CAD build for the part. Positions are in the model's coordinates, mm. A direction names the side the tool comes from. Round coordinates to 2 decimals unless told otherwise and drop trailing zeros. Write each loop counter-clockwise with the first axis right and the second up, starting at its lowest first coordinate (ties: lowest second). Pieces come first, ordered by that corner, then holes. Notation, with made-up numbers: M 27.5,-24 L 60.5,-24 A20 cw 60.5,10 Z; hole C 30.25,48 d4. An arc over 180 degrees is marked long. Write each question's results on one line, items separated by ' | '. Start each with the question number.
```python
from build123d import *

# Parameters (mm, degrees)
SKETCH1_W                = 44
SKETCH1_H                = 25
BOSS_EXTRUDE1_DEPTH      = 4.5
SKETCH2_W                = 44
SKETCH2_H                = 6
BOSS_EXTRUDE2_DEPTH      = 22
SKETCH3_R                = 1.6
SKETCH3_R_2              = 2.1
SKETCH3_R_3              = 3.1
SKETCH3_R_4              = 6.05
CUT_EXTRUDE1_DEPTH       = 34.529837459
SKETCH4_R                = 6.1
CUT_EXTRUDE2_DEPTH       = 0.7
SKETCH5_R                = 4.1
CUT_EXTRUDE3_DEPTH       = 0.5
SKETCH6_R                = 3.1
CUT_EXTRUDE4_DEPTH       = 0.4
CHAMFER4_SIZE            = 3
CHAMFER5_SIZE            = 2
CHAMFER6_SIZE            = 1.5
CHAMFER4_OF_MIRROR1_SIZE = 3
CHAMFER5_OF_MIRROR1_SIZE = 2
CHAMFER6_OF_MIRROR1_SIZE = 1.5
CUT_EXTRUDE5_DEPTH       = 43.558782877


with BuildPart() as part:
    # Sketch1 → Boss-Extrude1 (new body)
    with BuildSketch(Plane.XY):
        Rectangle(SKETCH1_W, SKETCH1_H)
    extrude(amount=BOSS_EXTRUDE1_DEPTH)

    # Sketch2 → Boss-Extrude2 (add)
    with BuildSketch(Plane.XY.offset(4.5)):
        with Locations((0, 9.5)):
            Rectangle(SKETCH2_W, SKETCH2_H)
    extrude(amount=BOSS_EXTRUDE2_DEPTH)

    # Sketch3 → Cut-Extrude1 (cut, through all)
    with BuildSketch(Plane.XY.offset(4.5)):
        with Locations((-14, -8.5)):
            Circle(SKETCH3_R)
        with Locations((-14, 0.682507664)):
            Circle(SKETCH3_R_2)
        with Locations((-3.234639789, -4.5)):
            Circle(SKETCH3_R_3)
        with Locations((12.315992983, -2.743651106)):
            Circle(SKETCH3_R_4)
    cut_extrude1 = extrude(amount=-CUT_EXTRUDE1_DEPTH, mode=Mode.SUBTRACT)

    # Sketch4 → Cut-Extrude2 (cut)
    with BuildSketch(Plane.XY.offset(4.5)):
        with Locations((-3.234639789, -4.5)):
            Circle(SKETCH4_R)
    cut_extrude2 = extrude(amount=-CUT_EXTRUDE2_DEPTH, mode=Mode.SUBTRACT)

    # Sketch5 → Cut-Extrude3 (cut)
    with BuildSketch(Plane.XY.offset(4.5)):
        with Locations((-14, 0.682507664)):
            Circle(SKETCH5_R)
    cut_extrude3 = extrude(amount=-CUT_EXTRUDE3_DEPTH, mode=Mode.SUBTRACT)

    # Sketch6 → Cut-Extrude4 (cut)
    with BuildSketch(Plane.XY.offset(4.5)):
        with Locations((-14, -8.5)):
            Circle(SKETCH6_R)
    cut_extrude4 = extrude(amount=-CUT_EXTRUDE4_DEPTH, mode=Mode.SUBTRACT)

    # Chamfer4
    chamfer4_edges = [part.edges().sort_by_distance(p)[0] for p in [
        (-6.334639789, -4.5, 3.8),
    ]]
    chamfer(chamfer4_edges, length=CHAMFER4_SIZE - 0.0001)  # a hair under: the kernel refuses the full size

    # Chamfer5
    chamfer5_edges = [part.edges().sort_by_distance(p)[0] for p in [
        (-16.1, 0.682507664, 4),
    ]]
    chamfer(chamfer5_edges, length=CHAMFER5_SIZE - 0.0001)  # a hair under: the kernel refuses the full size

    # Chamfer6
    chamfer6_edges = [part.edges().sort_by_distance(p)[0] for p in [
        (-15.6, -8.5, 4.1),
    ]]
    chamfer(chamfer6_edges, length=CHAMFER6_SIZE - 0.0001)  # a hair under: the kernel refuses the full size

    # Mirror1: Cut-Extrude1, Cut-Extrude2, Cut-Extrude3, Cut-Extrude4 across plane
    add(cut_extrude1.mirror(Plane(origin=(0, 5.5, 5.5), x_dir=(0, -0.7071067811865512, 0.7071067811865439), z_dir=(0, -0.7071067811865438, -0.7071067811865512))), mode=Mode.SUBTRACT)
    add(cut_extrude2.mirror(Plane(origin=(0, 5.5, 5.5), x_dir=(0, -0.7071067811865512, 0.7071067811865439), z_dir=(0, -0.7071067811865438, -0.7071067811865512))), mode=Mode.SUBTRACT)
    add(cut_extrude3.mirror(Plane(origin=(0, 5.5, 5.5), x_dir=(0, -0.7071067811865512, 0.7071067811865439), z_dir=(0, -0.7071067811865438, -0.7071067811865512))), mode=Mode.SUBTRACT)
    add(cut_extrude4.mirror(Plane(origin=(0, 5.5, 5.5), x_dir=(0, -0.7071067811865512, 0.7071067811865439), z_dir=(0, -0.7071067811865438, -0.7071067811865512))), mode=Mode.SUBTRACT)

    # Chamfer4 of Mirror1
    chamfer4_of_mirror1_edges = [part.edges().sort_by_distance(p)[0] for p in [
        (-6.334639789, 7.2, 15.5),
    ]]
    chamfer(chamfer4_of_mirror1_edges, length=CHAMFER4_OF_MIRROR1_SIZE - 0.0001)  # a hair under: the kernel refuses the full size

    # Chamfer5 of Mirror1
    chamfer5_of_mirror1_edges = [part.edges().sort_by_distance(p)[0] for p in [
        (-16.1, 7, 10.317492336),
    ]]
    chamfer(chamfer5_of_mirror1_edges, length=CHAMFER5_OF_MIRROR1_SIZE - 0.0001)  # a hair under: the kernel refuses the full size

    # Chamfer6 of Mirror1
    chamfer6_of_mirror1_edges = [part.edges().sort_by_distance(p)[0] for p in [
        (-15.6, 6.9, 19.5),
    ]]
    chamfer(chamfer6_of_mirror1_edges, length=CHAMFER6_OF_MIRROR1_SIZE - 0.0001)  # a hair under: the kernel refuses the full size

    # Sketch7 → Cut-Extrude5 (cut, through all)
    with BuildSketch(Plane(origin=(0, 12.5, 0), x_dir=(1, 0, 0), z_dir=(0, 1, 0))):
        Polygon((-14.3427417, -21.42), (-13.6572583, -21.42), (-12.86862915, -20.63137085), (-14, -19.5), (-15.13137085, -20.63137085), align=None)
        Polygon((-3.234639789, -15.5), (-1.042608767, -17.692031022), (-2.570577745, -19.22), (-3.898701832, -19.22), (-5.42667081, -17.692031022), align=None)
        Polygon((12.315992983, -13.743651106), (16.593989009, -18.021647132), (13.621985035, -20.993651106), (11.010000931, -20.993651106), (8.037996957, -18.021647132), align=None)
        Polygon((-14, -10.317492336), (-12.51507576, -11.802416576), (-13.550151519, -12.837492336), (-14.449848481, -12.837492336), (-15.48492424, -11.802416576), align=None)
    extrude(amount=-CUT_EXTRUDE5_DEPTH, mode=Mode.SUBTRACT)


solid = part.part
```
1) Drop flat-ended pins along their axis: pin 1 Ø1.9 at (x, z) = (-13, 20) entering from -Y; pin 2 Ø4 at (x, y) = (-17.5, -5) entering from +Z; pin 3 Ø11 at (x, z) = (-10, 20.5) entering from -Y; pin 4 Ø7.5 at (x, z) = (12.32, 13.74) entering from -Y. Give the stop position or say it passes through.
2) Saw through at D-D, the plane x = 10. Write the cut outline in (y, z), plus the area to 3 significant figures.
3) 3-axis set-ups, long thin cutter, end or side, ignore diameter. For faces 1 (the face through (-17.254, 6.746, 12.812)), 2 (the face through (-4.029, 1.548, 4.155)), 3 (the face through (-14, 11, 12.837)), 4 (the face through (-1.8, -7.25, 0.41)): which of +Z, -Z, +X, -X, +Y, -Y reach the whole face in a straight line?
4) Saw through at B-B, the plane y = -4.5. State how many separate pieces and enclosed holes the cut face has, plus the area to 3 significant figures.
5) Pull direction Z, two halves, no side cores. Call faces 5 (the face through (-16.1, 0.77, 1.01)), 6 (the face through (-1.72, 10.01, 12.58)), 7 (the face through (-1.467, -1.728, 0.988)): pulls with the +Z half, pulls with the -Z half, needs draft (parallel to the pull), parting line crosses it, or undercut.
6) Wall check: line 1 along Z through (x, y) = (-14, 11.15); line 2 along Z through (x, y) = (12, 11.5); line 3 along X through (y, z) = (-7.75, 1.5). Give the ranges that are in metal, low to high. Write a range as from..to.
7) Saw through at A-A, the plane x = 16. Write the cut outline in (y, z), plus the area to 3 significant figures.
Filled sheet:
1) pin 1: stops at y = 7.93 | pin 2: stops at z = 4.5 | pin 3: stops at y = 6.5 | pin 4: passes through
2) outline: M -12.5,0 L -8.33,0 L -8.33,4.5 L -12.5,4.5 Z; M 2.85,0 L 12.5,0 L 12.5,8.15 L 6.5,8.15 L 6.5,4.5 L 2.85,4.5 Z; M 6.5,19.98 L 12.5,19.98 L 12.5,26.5 L 6.5,26.5 Z | area: 123 mm^2
3) face 1: -Y | face 2: +Z | face 3: +Y, -Y | face 4: +Z, -Z
4) separate pieces: 3 | enclosed holes: 0 | area: 105 mm^2
5) face 5: needs draft | face 6: undercut | face 7: pulls with the +Z half
6) line 1: z = 0..8.22, 12.84..17.9, 21.42..26.5 | line 2: z = 0..7.7, 20.99..26.5 | line 3: x = -22..-15.41, -12.59..-5.2, -1.27..8.92, 15.71..22
7) outline: M -12.5,0 L -7.54,0 L -7.54,4.5 L -12.5,4.5 Z; M 2.06,0 L 12.5,0 L 12.5,8.94 L 6.5,8.94 L 6.5,4.5 L 2.06,4.5 Z; M 6.5,18.62 L 12.5,18.62 L 12.5,26.5 L 6.5,26.5 Z | area: 143 mm^2
